Read the model definition and answer for the solid it produces. Units are mm, in the model's axes. Face numbers are marked on the shaded views. A direction names the side the tool comes from. Round coordinates to 2 decimals unless told otherwise and drop trailing zeros. Order: outer loops, then holes, each group sorted by start corner. A loop starts at its lowest first (then second) coordinate and runs counter-clockwise, first axis right, second up. Notation, with made-up numbers: (26.5, -29) -> (43.5, -29) arc R23 ccw to (43.5, -8) -> close; hole circle Ø6 at (74, 4). An arc over 180 degrees is marked (long way). Answer as a JSON object with one key per item and string values. Group by question number.
Item 1: Given P1, Ø2, axis at x = 1, z = 28, coming from the +Y side; P2, Ø1.1, axis at y = 0.5, z = 31, coming from the -X side; P3, Ø1, axis at y = 1, z = 28.5, coming from the +X side, each flat-ended and moving along its own axis, determine where each tip first touches the part or whether it passes through.
Item 2: For the marked faces 4 and 5, determine the directions among +Z, -Z, +X, -X, +Y, -Y from which every point of the face is accessible in a straight line to the end or side of a thin tool.
Item 3: Section B-B, the plane z = 31.25 is taken. Write down the section's boundary in (x, y) (3 decimals), plus the area to 3 significant figures.
Item 4: The mould has two halves that part along X. Classify the marked faces 1, 2 and 3: pulls with the +X half, pulls with the -X half, needs draft (parallel to the pull), parting line crosses it, or undercut.
Item 5: Consider probe 1 along X at (y, z) = (0.1, 31) (3 decimals); probe 2 along Z at (x, y) = (1.1, -0.2); probe 3 along Y at (x, z) = (0, 29.75). Determine where each line is inside the solid, lowest interval first. Write a range as from..to.
Item 6: Section C-C, the plane z = 25.5 is taken. Write down the section's boundary in (x, y).
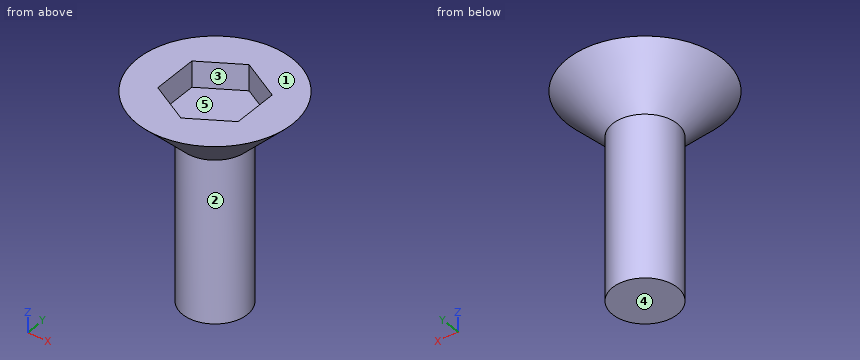
Solid Edge part; units mm, degrees
sketch "Sketch1" plane through (0, 0, 0) normal (0, 0, 1) x (1, 0, 0)
  circle A0 centre (0, 0) radius 1.25
extrude "Protrusion1" add sketch "Sketch1" along normal blind 30
sketch "Sketch2" plane through (0, 0, 30) normal (0, 0, 1) x (1, 0, 0)
  circle A0 centre (0, 0) radius 3
extrude "ExtrudedProtrusion_2" add sketch "Sketch2" along normal blind 1.75
chamfer "Chamfer_1" distance 1.75 angle 45 1 edges at (-3, 0, 30)
sketch "Sketch3" plane through (0, 0, 31.75) normal (0, 0, 1) x (0, 1, 0)
  line L0 (0.8978, -1.555) -> (1.7956, 0)
  line L1 (1.7956, 0) -> (0.8978, 1.555)
  line L2 (0.8978, 1.555) -> (-0.8978, 1.555)
  line L3 (-0.8978, 1.555) -> (-1.7956, 0)
  line L4 (-1.7956, 0) -> (-0.8978, -1.555)
  line L5 (-0.8978, -1.555) -> (0.8978, -1.555)
extrude "ExtrudedCutout_1" cut sketch "Sketch3" against normal blind 1
sketch "Sketch4" plane through (0, 0, 0) normal (0, 0, -1) x (0, 1, 0)
  circle A0 centre (0, 0) radius 1.9215
extrude "ExtrudedCutout_2" cut sketch "Sketch4" against normal blind 23.75
revolve "RevolvedCutout1" [suppressed]
fillet "Round_1" [suppressed]
properties material "Iron, grey cast type 20"
Values found:
{
 "1": {"P1": "y = 1.25", "P2": "x = -2.76", "P3": "x = 1.15"},
 "2": {"face 4": "-Z, +X, -X, +Y, -Y", "face 5": "+Z"},
 "3": {"outline": "circle Ø5 at (0, 0); hole (-1.555, -0.898) -> (0, -1.796) -> (1.555, -0.898) -> (1.555, 0.898) -> (0, 1.796) -> (-1.555, 0.898) -> close", "area": "11.3 mm2"},
 "4": {"face 1": "needs draft", "face 2": "parting line crosses it", "face 3": "undercut"},
 "5": {"probe 1": "-2.248..-1.555, 1.555..2.248", "probe 2": "23.75..30.75", "probe 3": "-1.25..1.25"},
 "6": {"outline": "circle Ø2.5 at (0, 0)"}
}
